Build history of the part. All positions in model axes, mm. Face numbers are marked on the shaded views. Round coordinates to 2 decimals unless told otherwise and drop trailing zeros. Write each loop counter-clockwise with the first axis right and the second up, starting at its lowest first coordinate (ties: lowest second). Pieces come first, ordered by that corner, then holes. Notation, with made-up numbers: (43, 63.25) -> (98, 63.25) arc R23 cw to (98, 102.25) -> close; hole circle Ø4 at (-11, 85). An arc over 180 degrees is marked (long way). Return JSON: item names as keys, results as strings.
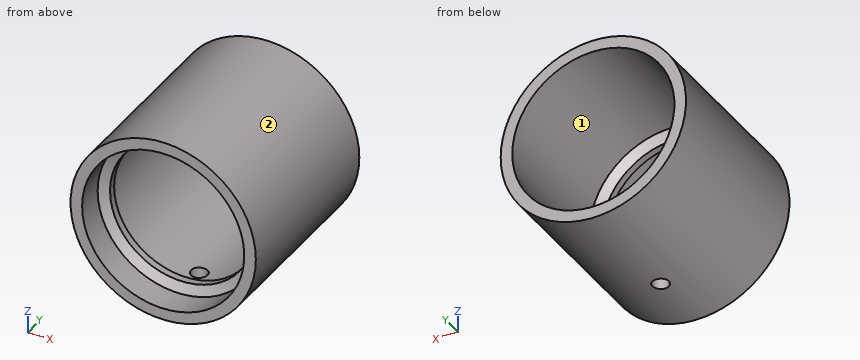
from build123d import *

# Parameters (mm, degrees)
F0_R      = 10
F1_DEPTH  = 20
F3_D      = 15.5
F5_D      = 17.5
F5_DEPTH  = 3
F5_TIP    = 5.2575304165
F7_D      = 17.5
F7_DEPTH  = 15
F7_TIP    = 5.2575304165
F10_D     = 1.778
F10_DEPTH = 12.9525
F10_START = 0.0395945
F10_TIP   = 0.5341650903


with BuildPart() as f1:
    # F0 (on Front) → F1 (new body)
    with BuildSketch(Plane.XZ):
        Circle(F0_R)
    extrude(amount=F1_DEPTH)

    # F3 (through all)
    with Locations(Plane(origin=(0, 0, 0), x_dir=(-1, 0, 0), z_dir=(0, 1, 0))):
        with Locations((0, 0)):
            Hole(F3_D / 2)

    # F5
    with Locations(Plane.XZ.offset(20)):
        with Locations((0, 0)):
            Hole(F5_D / 2, depth=F5_DEPTH)
            with Locations((0, 0, -(F5_DEPTH + F5_TIP / 2))):  # 118° drill point
                Cone(0, F5_D / 2, F5_TIP, mode=Mode.SUBTRACT)

    # F7
    with Locations(Plane(origin=(0, 0, 0), x_dir=(-1, 0, 0), z_dir=(0, 1, 0))):
        with Locations((0, 0)):
            Hole(F7_D / 2, depth=F7_DEPTH)
            with Locations((0, 0, -(F7_DEPTH + F7_TIP / 2))):  # 118° drill point
                Cone(0, F7_D / 2, F7_TIP, mode=Mode.SUBTRACT)

    # F10
    # its depths count from where the whole tool has entered the part; down to there all is cleared
    with Locations(Plane(origin=(0, 0, -10), x_dir=(1, 0, 0), z_dir=(0, 0, -1)).offset(-F10_START)):
        with Locations((0, 13)):
            Hole(F10_D / 2, depth=F10_DEPTH)
            with Locations((0, 0, -(F10_DEPTH + F10_TIP / 2))):  # 118° drill point
                Cone(0, F10_D / 2, F10_TIP, mode=Mode.SUBTRACT)


solid = f1.part
Q1. Saw through at B-B on y = -18.5. List the corners of the cut face in (x, z), then the cut area to 3 significant figures.
Verdict:
{"outline": "circle Ø20 at (0, 0); hole circle Ø17.5 at (0, 0)", "area": "73.6 mm²"}
Q2. Two-plate mould, pull along Z, no slides. Class the marked faces 1 and 2: +Z half, -Z half, draft (parallel to the pull), parting line (faces both ways), or undercut.
Verdict:
{"face 1": "undercut", "face 2": "parting line"}
Q3. Wall check: L1, parallel to Y at x = 0, z = -9.25; L2, parallel to Z at x = 0, y = -19; L3, parallel to Z at x = -5.25, y = -11.25. Give the ranges that are in metal, low to high.
Verdict:
{"L1": "y = -20 to -13.89, -12.11 to 0", "L2": "z = -10 to -8.75, 8.75 to 10", "L3": "z = -8.51 to -7, 7 to 8.51"}
Q4. Saw through at A-A on z = 0. List the corners of the cut face in (x, y).
Verdict:
{"outline": "(-10, -20) -> (-8.75, -20) -> (-8.75, -17) -> (-7.75, -16.4) -> (-7.75, -15.6) -> (-8.75, -15) -> (-8.75, 0) -> (-10, 0) -> close; (7.75, -16.4) -> (8.75, -17) -> (8.75, -20) -> (10, -20) -> (10, 0) -> (8.75, 0) -> (8.75, -15) -> (7.75, -15.6) -> close"}
Q5. Pin check, flat tips, straight feed: pin 1 Ø5 at (x, y) = (-6.5, -17.5) entering from +Z; pin 2 Ø4 at (y, z) = (-3, 5.5) entering from -X; pin 3 Ø1 at (y, z) = (-8.5, -7) entering from +X. Stop position of each tip, or through.
Verdict:
{"pin 1": "stops at z = 9.17", "pin 2": "stops at x = -9.37", "pin 3": "stops at x = 7.6"}
Q6. Saw through at C-C on y = -13. List the corners of the cut face in (x, z), then the cut area to 3 significant figures.
Verdict:
{"outline": "(-0.89, -9.96) -> (-0.89, -8.7) arc R8.75 cw (long way) to (0.89, -8.7) -> (0.89, -9.96) arc R10 ccw (long way) to start", "area": "71.4 mm²"}
